Check sheet for the modelled part. Datum: model origin and axes. Units: mm. A direction names the side the tool comes from. Coordinates: 2 decimals unless noted, no trailing zeros. Order: outer loops, then holes, each group sorted by start corner. A loop starts at its lowest first (then second) coordinate and runs counter-clockwise, first axis right, second up.
from build123d import *

# Parameters (mm, degrees)
F0_R     = 24.75
F0_R_2   = 22.75
F1_DEPTH = 1
F0_R_3   = 21.75
F0_R_4   = 20.75
F2_DEPTH = 8
F3_T     = 1


# Not quite as in the source:
# - a shell that OpenCascade refuses in one call is made with other operations: the cavity is built on its own and cut out


with BuildPart() as f1:
    # F0 (on Top) → F1 (new body)
    with BuildSketch(Plane.XY):
        with Locations((-30.0056487322, 13.6389313266)):
            Circle(F0_R)
        with Locations((-30.0056487322, 13.6389313266)):
            Circle(F0_R_2, mode=Mode.SUBTRACT)
    extrude(amount=F1_DEPTH)

    # F0 (on Top) → F2 (join)
    with BuildSketch(Plane.XY):
        with Locations((-30.0056487322, 13.6389313266)):
            Circle(F0_R_2)
        with Locations((-30.0056487322, 13.6389313266)):
            Circle(F0_R_3, mode=Mode.SUBTRACT)
        with Locations((-30.0056487322, 13.6389313266)):
            Circle(F0_R_3)
        with Locations((-30.0056487322, 13.6389313266)):
            Circle(F0_R_4, mode=Mode.SUBTRACT)
        with Locations((-30.0056487322, 13.6389313266)):
            Circle(F0_R_4)
    extrude(amount=F2_DEPTH)

    # F3: shell of thickness 1, made by hand


with BuildPart() as f3_core1:
    # F3_t2: copy of F1
    add(f1.part)

    # the walls: a layer under each face that stays
    f3_faces = [f3_core1.faces().sort_by_distance(p)[0] for p in [
        (-54.7556487322, 13.6389313266, 0.5),
        (-46.5056487322, -2.8610686734, 1),
        (-52.7556487322, 13.6389313266, 4.5),
        (-30.0056487322, 13.6389313266, 8),
    ]]
    thicken(f3_faces, amount=-F3_T, mode=Mode.SUBTRACT)

    # F3_s3 → F3_t4 (revolve, cut)
    with BuildSketch(Plane.XZ.offset(-13.6389313266)):
        Polygon((-7.2456487322, 1.01), (-7.2556487322, 0), (-8.2556487322, 0), (-8.2556487322, 1), align=None)
    revolve(axis=Axis((-30.0056487322, 13.6389313266, 1), (0, 0, 1)), mode=Mode.SUBTRACT)


with BuildPart() as f1_1:
    add(f1.part)

    # what is left inside the walls is the cavity
    f3_cavity = [f3_core1.part.solids().sort_by_distance(p)[0] for p in [
        (-30.005649, 6.388931, 6.99),
    ]]
    add(f3_cavity, mode=Mode.SUBTRACT)


solid = f1_1.part
(1) Go/stop test with flat-tipped pins: P1, Ø3, axis at x = -39, y = -3, coming from the -Z side; P2, Ø1.5, axis at y = -1.5, z = 6.5, coming from the -X side; P3, Ø4, axis at x = -44.5, z = 2.5, coming from the +Y side. Record where each tip stops, or that it passes through.
Filled in:
P1: stops at z = 7
P2: stops at x = -47.63
P3: stops at y = 34.59
(2) Tool access check on faces 5 (the flat face through (-8, 6, 1)), 6 (the cylindrical face through (-7.143, 4.16, 0.493)). Record the directions out of +Z, -Z, +X, -X, +Y, -Y that give a thin tool (end or side, any length) a straight path to the whole face; none if there is none.
Filled in:
face 5: +Z
face 6: +Z, -Z
(3) Cross-section at B-B (x = -27). Enter the section's corners in (y, z), and give its area (3 significant figures).
Filled in:
outline: (-10.93, 0) - (-7.9, 0) - (-7.9, 7) - (35.18, 7) - (35.18, 0) - (38.21, 0) - (38.21, 1) - (36.19, 1) - (36.19, 8) - (-8.91, 8) - (-8.91, 1) - (-10.93, 1) - close
area: 63.3 mm2
(4) Thickness scan on probe 1 along Z at (x, y) = (-30.5, -6); probe 2 along X at (y, z) = (17, 3.5); probe 3 along X at (y, z) = (11, 3.5). Record the ranges inside material, lowest first.
Filled in:
probe 1: z = 7 to 8
probe 2: x = -52.51 to -51.49, -8.52 to -7.51
probe 3: x = -52.6 to -51.59, -8.42 to -7.41
(5) Cross-section at C-C (z = 2.5). Enter the section's corners in (x, y), and give its area (3 significant figures).
Filled in:
outline: circle Ø45.5 at (-30.01, 13.64); hole circle Ø43.5 at (-30.01, 13.64)
area: 140 mm2
(6) Release check for a two-part mould opening along Y. For faces 1 (the flat face through (-28.3, -8.2, 0)), 2 (the cylindrical face through (-47.266, 0.404, 3.549)), 3 (the flat face through (-30, 14, 7)), 4 (the cylindrical face through (-48.06, -0.2, 4.45)) record: +Y half, -Y half, draft (parallel to the pull), parting line (faces both ways), or undercut.
Filled in:
face 1: draft
face 2: undercut
face 3: undercut
face 4: parting line
(7) Cross-section at A-A (y = 25.5). Enter the section's corners in (x, z).
Filled in:
outline: (-51.73, 0) - (-48.24, 0) - (-48.24, 7) - (-11.77, 7) - (-11.77, 0) - (-8.28, 0) - (-8.28, 1) - (-10.59, 1) - (-10.59, 8) - (-49.42, 8) - (-49.42, 1) - (-51.73, 1) - close
